Read the model definition and answer for the solid it produces. Units are mm, in the model's axes. A direction names the side the tool comes from. Coordinates: 2 decimals unless noted, no trailing zeros. Write each loop counter-clockwise with the first axis right and the second up, starting at its lowest first coordinate (ties: lowest second). Pieces come first, ordered by that corner, then holes. Notation, with made-up numbers: (38, 30.5) -> (72, 30.5) arc R15 ccw to (72, 55.5) -> close; hole circle Ø4 at (73.25, -19). An arc over 180 degrees is marked (long way). Return JSON: item names as keys, results as strings.
from build123d import *

# Parameters (mm, degrees)
SKETCH1_R                = 19.05
BOSS_EXTRUDE1_DEPTH      = 127
BOSS_EXTRUDE2_DEPTH      = 12.7
BOSS_EXTRUDE3_DEPTH      = 12.7
BOSS_EXTRUDE3_DEPTH_BACK = 38.1
SKETCH1_4_R              = 9.525
BOSS_EXTRUDE4_START      = -38.1
BOSS_EXTRUDE4_DEPTH      = 12.7
BOSS_EXTRUDE5_START      = -88.9
SKETCH1_6_R              = 9.525
BOSS_EXTRUDE5_DEPTH      = 63.5
BOSS_EXTRUDE6_START      = -88.9
BOSS_EXTRUDE6_DEPTH      = 12.7
BOSS_EXTRUDE7_START      = -114.3
SKETCH1_8_R              = 9.525
BOSS_EXTRUDE7_DEPTH      = 38.1


with BuildPart() as part:
    # Sketch1 → Boss-Extrude1 (new body)
    with BuildSketch(Plane(origin=(0, 0, 0), x_dir=(0, 0, -1), z_dir=(1, 0, 0))):
        Circle(SKETCH1_R)
    extrude(amount=BOSS_EXTRUDE1_DEPTH)

    # Sketch1_3 → Boss-Extrude2 (add)
    with BuildSketch(Plane(origin=(0, 0, 0), x_dir=(0, 0, -1), z_dir=(1, 0, 0))):
        with BuildLine():
            ThreePointArc((76.2, -9.525), (66.675, 0), (76.2, 9.525))
            Line((76.2, 9.525), (16.497783942, 9.525))
            ThreePointArc((16.497783942, 9.525), (18.400886991, 4.930502809), (19.05, 0))
            ThreePointArc((19.05, 0), (18.400886991, -4.930502809), (16.497783942, -9.525))
            Line((16.497783942, -9.525), (76.2, -9.525))
        make_face()
    extrude(amount=BOSS_EXTRUDE2_DEPTH)

    # Sketch1_4 → Boss-Extrude3 (add, two sides: drawn at the far end of the back side and taken through both)
    with BuildSketch(Plane(origin=(0, 0, 0), x_dir=(0, 0, -1), z_dir=(1, 0, 0)).offset(-BOSS_EXTRUDE3_DEPTH_BACK)):
        with Locations((76.2, 0)):
            Circle(SKETCH1_4_R)
    extrude(amount=BOSS_EXTRUDE3_DEPTH + BOSS_EXTRUDE3_DEPTH_BACK)

    # Sketch1_5 → Boss-Extrude4 (add)
    with BuildSketch(Plane(origin=(0, 0, 0), x_dir=(0, 0, -1), z_dir=(1, 0, 0)).offset(BOSS_EXTRUDE4_START)):
        with BuildLine():
            ThreePointArc((127, -9.525), (117.475, 0), (127, 9.525))
            Line((127, 9.525), (76.2, 9.525))
            ThreePointArc((76.2, 9.525), (82.935192091, 6.735192091), (85.725, 0))
            ThreePointArc((85.725, 0), (82.935192091, -6.735192091), (76.2, -9.525))
            Line((76.2, -9.525), (127, -9.525))
        make_face()
    extrude(amount=BOSS_EXTRUDE4_DEPTH)

    # Sketch1_6 → Boss-Extrude5 (add)
    with BuildSketch(Plane(origin=(0, 0, 0), x_dir=(0, 0, -1), z_dir=(1, 0, 0)).offset(BOSS_EXTRUDE5_START)):
        with Locations((127, 0)):
            Circle(SKETCH1_6_R)
    extrude(amount=BOSS_EXTRUDE5_DEPTH)

    # Sketch1_7 → Boss-Extrude6 (add)
    with BuildSketch(Plane(origin=(0, 0, 0), x_dir=(0, 0, -1), z_dir=(1, 0, 0)).offset(BOSS_EXTRUDE6_START)):
        with BuildLine():
            ThreePointArc((127, -9.525), (117.475, 0), (127, 9.525))
            Line((127, 9.525), (76.2, 9.525))
            ThreePointArc((76.2, 9.525), (82.935192091, 6.735192091), (85.725, 0))
            ThreePointArc((85.725, 0), (82.935192091, -6.735192091), (76.2, -9.525))
            Line((76.2, -9.525), (127, -9.525))
        make_face()
    extrude(amount=BOSS_EXTRUDE6_DEPTH)

    # Sketch1_8 → Boss-Extrude7 (add)
    with BuildSketch(Plane(origin=(0, 0, 0), x_dir=(0, 0, -1), z_dir=(1, 0, 0)).offset(BOSS_EXTRUDE7_START)):
        with Locations(Location((76.2, 0, 0), (0, 0, 90))):
            Circle(SKETCH1_8_R)
    extrude(amount=BOSS_EXTRUDE7_DEPTH)


solid = part.part
1. For a pull along X with two mould halves and no side action, classify faces 1 (the face through (6, -9.525, -46)), 2 (the face through (-38.1, 0, -96)), 3 (the face through (0, 0, -17)) as +X half, -X half, draft (parallel to the pull), parting line (faces both ways), or undercut.
Taken from the geometry:
{"face 1": "draft", "face 2": "undercut", "face 3": "-X half"}
2. The part is cut by section D-D (z = -81.5). Determine the outline of the cut face in (x, y) (3 decimals), then the cut area to 3 significant figures.
Taken from the geometry:
{"outline": "(-114.3, -7.914) -> (-88.9, -7.914) -> (-88.9, -9.525) -> (-76.2, -9.525) -> (-76.2, 9.525) -> (-88.9, 9.525) -> (-88.9, 7.914) -> (-114.3, 7.914) -> close; (-38.1, -9.525) -> (-25.4, -9.525) -> (-25.4, -7.914) -> (12.7, -7.914) -> (12.7, 7.914) -> (-25.4, 7.914) -> (-25.4, 9.525) -> (-38.1, 9.525) -> close", "area": "1,490 mm2"}
3. The part is cut by section C-C (x = 8.5). Determine the outline of the cut face in (y, z) (3 decimals), then the cut area to 3 significant figures.
Taken from the geometry:
{"outline": "(-9.525, -76.2) arc R9.525 ccw to (9.525, -76.2) -> (9.525, -16.498) arc R19.05 ccw (long way) to (-9.525, -16.498) -> close", "area": "2,390 mm2"}
4. The part is cut by section A-A (z = -101). Determine the outline of the cut face in (x, y) (3 decimals), then the cut area to 3 significant figures.
Taken from the geometry:
{"outline": "(-88.9, -9.525) -> (-76.2, -9.525) -> (-76.2, 9.525) -> (-88.9, 9.525) -> close; (-38.1, -9.525) -> (-25.4, -9.525) -> (-25.4, 9.525) -> (-38.1, 9.525) -> close", "area": "484 mm2"}
5. Consider L1, parallel to X at y = -3.5, z = -76; L2, parallel to X at y = 9, z = -100.5; L3, parallel to X at y = 4, z = -30.5. Determine where each line is inside the solid, lowest interval first.
Taken from the geometry:
{"L1": "x = -114.3 to -76.2, -38.1 to 12.7", "L2": "x = -88.9 to -76.2, -38.1 to -25.4", "L3": "x = 0 to 12.7"}
6. A tool of negligible diameter and unlimited length cuts with its end or side. For faces 4 (the face through (6, 9.525, -47)), 5 (the face through (-13.056, 2.861, -85.285)), 6 (the face through (-99.75, -1.24, -66.756)), 7 (the face through (-83, 9.525, -102)), 8 (the face through (62.61, 0.84, 19.03)), from which of +Z, -Z, +X, -X, +Y, -Y can it reach the whole face along a straight path? Write none if from no direction.
Taken from the geometry:
{"face 4": "-Z, +X, -X, +Y", "face 5": "none", "face 6": "-X", "face 7": "+Z, -Z, +X, -X, +Y", "face 8": "+X"}
7. Flat-ended cylindrical pins translate along their axes: pin 1 Ø1 at (x, y) = (93, -11.5) entering from +Z; pin 2 Ø5.5 at (y, z) = (4.5, -90) entering from +X; pin 3 Ø12 at (y, z) = (13, -117.5) entering from -X; pin 4 Ø12 at (x, z) = (19, -51.5) entering from -Y. Find the tip coordinate at first contact, or state that the pin passes through.
Taken from the geometry:
{"pin 1": "stops at z = 15.55", "pin 2": "stops at x = -25.4", "pin 3": "stops at x = -88.9", "pin 4": "passes through"}
8. The part is cut by section B-B (y = 0). Determine the outline of the cut face in (x, z) (3 decimals), then the cut area to 3 significant figures.
Taken from the geometry:
{"outline": "(-114.3, -85.725) -> (-88.9, -85.725) -> (-88.9, -136.525) -> (-25.4, -136.525) -> (-25.4, -85.725) -> (12.7, -85.725) -> (12.7, -19.05) -> (127, -19.05) -> (127, 19.05) -> (0, 19.05) -> (0, -66.675) -> (-38.1, -66.675) -> (-38.1, -117.475) -> (-76.2, -117.475) -> (-76.2, -66.675) -> (-114.3, -66.675) -> close", "area": "9,150 mm2"}
